from build123d import *

# Parameters (mm, degrees)
SKETCH1_W           = 81.3
SKETCH1_H           = 46
BOSS_EXTRUDE1_DEPTH = 3
SKETCH5_W           = 3
SKETCH5_H           = 5
BOSS_EXTRUDE3_DEPTH = 5
SKETCH6_R           = 1.5
CUT_EXTRUDE2_DEPTH  = 47.972571784
FILLET5_RADIUS      = 2.5
FILLET5_LENGTH      = 3
SKETCH7_R           = 1.5
CUT_EXTRUDE3_DEPTH  = 10


with BuildPart() as part:
    # Sketch1 → Boss-Extrude1 (new body)
    with BuildSketch(Plane.XY):
        Rectangle(SKETCH1_W, SKETCH1_H)
    extrude(amount=-BOSS_EXTRUDE1_DEPTH)

    # Sketch5 → Boss-Extrude3 (add)
    with BuildSketch(Plane.XY):
        with Locations((35.65, 0)):
            Rectangle(SKETCH5_W, SKETCH5_H)
    extrude(amount=BOSS_EXTRUDE3_DEPTH)

    # Sketch6 → Cut-Extrude2 (cut, through all)
    with BuildSketch(Plane(origin=(0, 0, 0), x_dir=(0, 0, -1), z_dir=(1, 0, 0))):
        with Locations(Location((-2.5, 0, 0), (0, 0, 180))):
            Circle(SKETCH6_R)
    extrude(amount=CUT_EXTRUDE2_DEPTH, mode=Mode.SUBTRACT)

    # Fillet5: full round fillet: the end face becomes a half cylinder, R = half its width
    fillet5_face = Plane((35.65, 0, 5), x_dir=(-1, 0, 0), z_dir=(0, 0, 1))  # on the end face: x along it, z out of the body
    fillet5_slab = fillet5_face.offset(-FILLET5_RADIUS / 2) * Box(FILLET5_LENGTH, 2 * FILLET5_RADIUS, FILLET5_RADIUS, mode=Mode.PRIVATE)  # the body's end, R deep
    fillet5_round = Plane((35.65, 0, 2.5), x_dir=(0, 0, 1), z_dir=(-1, 0, 0)) * Cylinder(FILLET5_RADIUS, FILLET5_LENGTH, mode=Mode.PRIVATE)  # its axis R under the face
    add(fillet5_slab - fillet5_round, mode=Mode.SUBTRACT)

    # Sketch7 → Cut-Extrude3 (cut)
    with BuildSketch(Plane.XY):
        with Locations((-34.55, -9)):
            Circle(SKETCH7_R)
        with Locations((-34.55, 6)):
            Circle(SKETCH7_R)
    extrude(amount=-CUT_EXTRUDE3_DEPTH, mode=Mode.SUBTRACT)


solid = part.part
Work out the finished part from the listing and answer in its coordinate system (mm). A direction names the side the tool comes from. Coordinates: 2 decimals unless noted, no trailing zeros. Write each loop counter-clockwise with the first axis right and the second up, starting at its lowest first coordinate (ties: lowest second). Pieces come first, ordered by that corner, then holes.
1. The part is cut by section D-D, the plane x = 5. Write down the section's boundary in (y, z).
Results list:
outline: (-23, -3) - (23, -3) - (23, 0) - (-23, 0) - close
2. For a pull along X with two mould halves and no side action, classify faces 1 (the cylindrical face through (-35.74, -9.91, -1.48)), 2 (the cylindrical face through (-35.74, 5.09, -1.48)), 3 (the flat face through (36, -2.5, 1)), 4 (the flat face through (37.15, 1, 1)) as +X half, -X half, draft (parallel to the pull), parting line (faces both ways), or undercut.
Results list:
face 1: undercut
face 2: undercut
face 3: draft
face 4: +X half
3. The part is cut by section C-C, the plane y = -9. Write down the section's boundary in (x, z), and give its area (3 significant figures).
Results list:
outline: (-40.65, -3) - (-36.05, -3) - (-36.05, 0) - (-40.65, 0) - close; (-33.05, -3) - (40.65, -3) - (40.65, 0) - (-33.05, 0) - close
area: 235 mm2
4. The part is cut by section B-B, the plane y = 0. Write down the section's boundary in (x, z).
Results list:
outline: (-40.65, -3) - (40.65, -3) - (40.65, 0) - (37.15, 0) - (37.15, 1) - (34.15, 1) - (34.15, 0) - (-40.65, 0) - close; (34.15, 4) - (37.15, 4) - (37.15, 5) - (34.15, 5) - close
5. Consider line 1 along Y through (x, z) = (-34.55, -1.65); line 2 along Y through (x, z) = (35.95, 2.5); line 3 along Z through (x, y) = (13, -11). Determine where each line is inside the solid, lowest interval first.
Results list:
line 1: y = -23 to -10.5, -7.5 to 4.5, 7.5 to 23
line 2: y = -2.5 to -1.5, 1.5 to 2.5
line 3: z = -3 to 0
6. For faces 5 (the flat face through (36, 2.5, 1)), 6 (the flat face through (-1, 23, -1)), 7 (the flat face through (34.15, 1, 1)), determine the directions among +Z, -Z, +X, -X, +Y, -Y from which every point of the face is accessible in a straight line to the end or side of a thin tool.
Results list:
face 5: +Z, +X, -X, +Y
face 6: +Z, -Z, +X, -X, +Y
face 7: +Z, -X, +Y, -Y
7. Flat-ended cylindrical pins translate along their axes: pin 1 (3.5 mm diameter, centred on y = 0, z = 2.5, fed in from +X); pin 2 (1.5 mm diameter, centred on x = -27, y = 11.5, fed in from +Z); pin 3 (2 mm diameter, centred on x = 36, z = 2, fed in from -Y). Find the tip coordinate at first contact, or state that the pin passes through.
Results list:
pin 1: stops at x = 37.15
pin 2: stops at z = 0
pin 3: stops at y = -2.5
8. The part is cut by section A-A, the plane x = -34.55. Write down the section's boundary in (y, z), and give its area (3 significant figures).
Results list:
outline: (-23, -3) - (-10.5, -3) - (-10.5, 0) - (-23, 0) - close; (-7.5, -3) - (4.5, -3) - (4.5, 0) - (-7.5, 0) - close; (7.5, -3) - (23, -3) - (23, 0) - (7.5, 0) - close
area: 120 mm2
